```python
from build123d import *

# Parameters (mm, degrees)
F1_DEPTH  = 50
F2_R      = 3
F3_DEPTH  = 2.5
F5_DEPTH  = 3
F7_DEPTH  = 3
F8_W      = 40
F8_H      = 2.5
F9_DEPTH  = 40
F10_DEPTH = 25


with BuildPart() as f1:
    # F0 (on Top) → F1 (new body)
    with BuildSketch(Plane.XY):
        Polygon((-2.5, 0), (0, 0), (0, 350), (-220, 350), (-220, 385), (-222.5, 385), (-222.5, 347.5), (-2.5, 347.5), align=None)
        Polygon((0, -350), (0, 0), (-2.5, 0), (-2.5, -347.5), (-222.5, -347.5), (-222.5, -385), (-220, -385), (-220, -350), align=None)
    extrude(amount=F1_DEPTH)

    # F2 (on Right) → F3 (join)
    with BuildSketch(Plane.YZ):
        Polygon((20, 0), (0, 0), (-20, 0), (-20, -40), (20, -40), align=None)
        with Locations((0, -30)):
            Circle(F2_R, mode=Mode.SUBTRACT)
        with Locations((0, -15)):
            Circle(F2_R, mode=Mode.SUBTRACT)
    extrude(amount=-F3_DEPTH)

    # F4 (on face) → F5 (cut)
    with BuildSketch(Plane.YZ.offset(-220)):
        with BuildLine():
            Line((-367.324291, 39.496568), (-367.682109, 39.496314))
            ThreePointArc((-367.682109, 39.496314), (-371.999078, 34.908927), (-367.5, 30.5))
            ThreePointArc((-367.5, 30.5), (-366.193757, 30.693757), (-365, 31.258343))
            ThreePointArc((-365, 31.258343), (-366.468627, 32.87868), (-367, 35))
            ThreePointArc((-367, 35), (-366.468627, 37.12132), (-365, 38.741657))
            ThreePointArc((-365, 38.741657), (-366.109918, 39.279915), (-367.324291, 39.496568))
        make_face()
        with BuildLine():
            ThreePointArc((-367.324291, 39.496568), (-367.503202, 39.499999), (-367.682109, 39.496314))
            Line((-367.682109, 39.496314), (-367.324291, 39.496568))
        make_face()
        with BuildLine():
            ThreePointArc((-365, 31.258343), (-366.193757, 30.693757), (-367.5, 30.5))
            Line((-367.5, 30.5), (-362.5, 30.5))
            ThreePointArc((-362.5, 30.5), (-363.806243, 30.693757), (-365, 31.258343))
        make_face()
        with BuildLine():
            Line((-362.503202, 39.499999), (-367.324291, 39.496568))
            ThreePointArc((-367.324291, 39.496568), (-366.109918, 39.279915), (-365, 38.741657))
            ThreePointArc((-365, 38.741657), (-363.807775, 39.305778), (-362.503202, 39.499999))
        make_face()
        with BuildLine():
            ThreePointArc((-363, 35), (-363.531373, 32.87868), (-365, 31.258343))
            ThreePointArc((-365, 31.258343), (-363.806243, 30.693757), (-362.5, 30.5))
            ThreePointArc((-362.5, 30.5), (-359.318019, 31.818019), (-358, 35))
            ThreePointArc((-358, 35), (-359.319152, 38.183112), (-362.503202, 39.499999))
            ThreePointArc((-362.503202, 39.499999), (-363.807775, 39.305778), (-365, 38.741657))
            ThreePointArc((-365, 38.741657), (-363.531373, 37.12132), (-363, 35))
        make_face()
        with BuildLine():
            ThreePointArc((-365, 18.741657), (-366.188395, 19.304613), (-367.488792, 19.499986))
            ThreePointArc((-367.488792, 19.499986), (-371.999046, 15.092651), (-367.674064, 10.503368))
            Line((-367.674064, 10.503368), (-367.325936, 10.503368))
            ThreePointArc((-367.325936, 10.503368), (-366.110701, 10.719831), (-365, 11.258343))
            ThreePointArc((-365, 11.258343), (-366.468627, 12.87868), (-367, 15))
            ThreePointArc((-367, 15), (-366.468627, 17.12132), (-365, 18.741657))
        make_face()
        with BuildLine():
            Line((-362.500013, 19.5), (-367.488792, 19.499986))
            ThreePointArc((-367.488792, 19.499986), (-366.188395, 19.304613), (-365, 18.741657))
            ThreePointArc((-365, 18.741657), (-363.806249, 19.306241), (-362.500013, 19.5))
        make_face()
        with BuildLine():
            Line((-367.325936, 10.503368), (-367.674064, 10.503368))
            ThreePointArc((-367.674064, 10.503368), (-367.5, 10.5), (-367.325936, 10.503368))
        make_face()
        with BuildLine():
            ThreePointArc((-362.500013, 19.5), (-363.806249, 19.306241), (-365, 18.741657))
            ThreePointArc((-365, 18.741657), (-363.531373, 17.12132), (-363, 15))
            ThreePointArc((-363, 15), (-363.531373, 12.87868), (-365, 11.258343))
            ThreePointArc((-365, 11.258343), (-363.889299, 10.719831), (-362.674064, 10.503368))
            Line((-362.674064, 10.503368), (-362.325936, 10.503368))
            ThreePointArc((-362.325936, 10.503368), (-359.257062, 11.880167), (-358, 15))
            ThreePointArc((-358, 15), (-359.318024, 18.181985), (-362.500013, 19.5))
        make_face()
        with BuildLine():
            ThreePointArc((-365, 11.258343), (-366.110701, 10.719831), (-367.325936, 10.503368))
            Line((-367.325936, 10.503368), (-362.674064, 10.503368))
            ThreePointArc((-362.674064, 10.503368), (-363.889299, 10.719831), (-365, 11.258343))
        make_face()
        with BuildLine():
            Line((-362.325936, 10.503368), (-362.674064, 10.503368))
            ThreePointArc((-362.674064, 10.503368), (-362.5, 10.5), (-362.325936, 10.503368))
        make_face()
        with BuildLine():
            ThreePointArc((-363, 35), (-363.531373, 37.12132), (-365, 38.741657))
            ThreePointArc((-365, 38.741657), (-366.468627, 37.12132), (-367, 35))
            Line((-367, 35), (-363, 35))
        make_face()
        with BuildLine():
            ThreePointArc((-365, 11.258343), (-363.531373, 12.87868), (-363, 15))
            Line((-363, 15), (-367, 15))
            ThreePointArc((-367, 15), (-366.468627, 12.87868), (-365, 11.258343))
        make_face()
        with BuildLine():
            ThreePointArc((-363, 15), (-363.531373, 17.12132), (-365, 18.741657))
            ThreePointArc((-365, 18.741657), (-366.468627, 17.12132), (-367, 15))
            Line((-367, 15), (-363, 15))
        make_face()
        with BuildLine():
            ThreePointArc((-367, 35), (-366.468627, 32.87868), (-365, 31.258343))
            ThreePointArc((-365, 31.258343), (-363.531373, 32.87868), (-363, 35))
            Line((-363, 35), (-367, 35))
        make_face()
    extrude(amount=-F5_DEPTH, mode=Mode.SUBTRACT)

    # F6 (on face) → F7 (cut)
    with BuildSketch(Plane.YZ.offset(-220)):
        with BuildLine():
            Line((362.951623, 30.52272), (367.951623, 30.52272))
            ThreePointArc((367.951623, 30.52272), (372, 35), (367.951623, 39.47728))
            Line((367.951623, 39.47728), (362.951623, 39.47728))
            ThreePointArc((362.951623, 39.47728), (358, 35), (362.951623, 30.52272))
        make_face()
        with BuildLine():
            Line((368.176887, 10.5512), (366.903754, 10.539676))
            ThreePointArc((366.903754, 10.539676), (367.54073, 10.500184), (368.176887, 10.5512))
        make_face()
        with BuildLine():
            Line((362.54073, 10.500184), (366.903754, 10.539676))
            Line((366.903754, 10.539676), (368.176887, 10.5512))
            ThreePointArc((368.176887, 10.5512), (372, 15), (368.176887, 19.4488))
            Line((368.176887, 19.4488), (362.54073, 19.499816))
            ThreePointArc((362.54073, 19.499816), (358, 15), (362.54073, 10.500184))
        make_face()
    extrude(amount=-F7_DEPTH, mode=Mode.SUBTRACT)

    # F8 (on face) → F9 (join)
    with BuildSketch(Plane.YZ):
        with Locations((0, -38.75)):
            Rectangle(F8_W, F8_H)
    extrude(amount=-F9_DEPTH)

    # F6 (on face) → F10 (cut)
    with BuildSketch(Plane.YZ.offset(-220)):
        with BuildLine():
            Line((362.951623, 30.52272), (367.951623, 30.52272))
            ThreePointArc((367.951623, 30.52272), (372, 35), (367.951623, 39.47728))
            Line((367.951623, 39.47728), (362.951623, 39.47728))
            ThreePointArc((362.951623, 39.47728), (358, 35), (362.951623, 30.52272))
        make_face()
        with BuildLine():
            Line((368.176887, 10.5512), (366.903754, 10.539676))
            ThreePointArc((366.903754, 10.539676), (367.54073, 10.500184), (368.176887, 10.5512))
        make_face()
        with BuildLine():
            Line((362.54073, 10.500184), (366.903754, 10.539676))
            Line((366.903754, 10.539676), (368.176887, 10.5512))
            ThreePointArc((368.176887, 10.5512), (372, 15), (368.176887, 19.4488))
            Line((368.176887, 19.4488), (362.54073, 19.499816))
            ThreePointArc((362.54073, 19.499816), (358, 15), (362.54073, 10.500184))
        make_face()
    extrude(amount=-F10_DEPTH, mode=Mode.SUBTRACT)


solid = f1.part
```
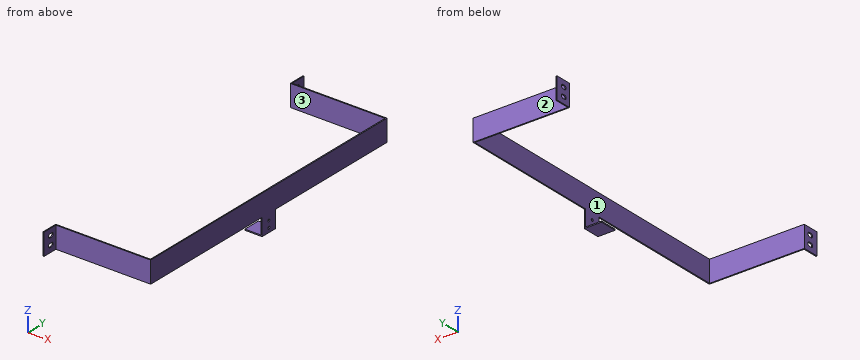
Input: part model. Units: mm. Frame: model coordinates. Face numbers are marked on the shaded views. A direction names the side the tool comes from. Coordinates: 2 decimals unless noted, no trailing zeros. Loops run counter-clockwise (first coordinate to the right, second up) from the corner with the lowest first, then second, coordinate; pieces in that order, holes last. Notation, with made-up numbers: (28, 63.5) -> (86, 63.5) arc R21 cw to (86, 102.5) -> close; hole circle Ø2 at (33, -35.5). An arc over 180 degrees is marked (long way). Use a Markdown table: item, result.
1) Cut plane B-B (y = 144.5). Return the cut outline in (x, z), then the cut area to 3 significant figures.
Results found:
| item | result |
|---|---|
| outline | (-2.5, 0) -> (0, 0) -> (0, 50) -> (-2.5, 50) -> close |
| area | 125 mm2 |
2) Access query for the marked faces 1, 2 and 3. Directions: +Z, -Z, +X, -X, +Y, -Y. A direction counts if a zero-diameter tool reaches every point of the face in a straight line with its end or side. Return the directions, or none.
Results found:
| item | result |
|---|---|
| face 1 | +Z, -X |
| face 2 | +Z, -Z, +X, +Y |
| face 3 | +Z, -Z, -X |
3) Contact query for flat-ended pins moving along their axis: pin 1 (1.2 mm diameter, centred on y = -2.5, z = -39, fed in from -X); pin 2 (12 mm diameter, centred on x = -181.5, z = 33.5, fed in from +Y); pin 3 (17.5 mm diameter, centred on y = -370.5, z = 36.5, fed in from +X). Output: stop coordinate, or through.
Results found:
| item | result |
|---|---|
| pin 1 | stops at x = -40 |
| pin 2 | stops at y = 350 |
| pin 3 | stops at x = -220 |
4) Cut plane A-A (x = -197). Return the cut outline in (y, z).
Results found:
| item | result |
|---|---|
| outline | (-350, 0) -> (-347.5, 0) -> (-347.5, 50) -> (-350, 50) -> close; (347.5, 0) -> (350, 0) -> (350, 50) -> (347.5, 50) -> close |
5) Material intervals for line 1 along Z through (x, y) = (-1.8, 0); line 2 along Y through (x, z) = (-29.5, 16); line 3 along X through (y, z) = (195, 38), sorted ascending. Write a range as from..to.
Results found:
| item | result |
|---|---|
| line 1 | z = -40..-33, -27..-18, -12..50 |
| line 2 | y = -350..-347.5, 347.5..350 |
| line 3 | x = -2.5..0 |
